```python
from build123d import *

# Parameters (mm, degrees)
BOSS_EXTRUDE1_DEPTH = 100
SKETCH2_R           = 2.75
CUT_EXTRUDE1_DEPTH  = 100
CUT_EXTRUDE2_DEPTH  = 100


with BuildPart() as part:
    # Sketch1 → Boss-Extrude1 (new body)
    with BuildSketch(Plane.XY):
        Polygon((0, 0), (-60, 0), (-60, -50), (-57, -50), (-57, -3), (0, -3), align=None)
    extrude(amount=BOSS_EXTRUDE1_DEPTH)

    # Sketch2 → Cut-Extrude1 (cut)
    with BuildSketch(Plane(origin=(0, 0, 0), x_dir=(1, 0, 0), z_dir=(0, 1, 0))):
        with Locations(Location((-11.813466521, -80.5, 0), (0, 0, 180))):
            Circle(SKETCH2_R)
        with Locations(Location((-48.186533479, -80.5, 0), (0, 0, 180))):
            Circle(SKETCH2_R)
        with Locations(Location((-30, -49, 0), (0, 0, 180))):
            Circle(SKETCH2_R)
    extrude(amount=-CUT_EXTRUDE1_DEPTH, mode=Mode.SUBTRACT)

    # Sketch3 → Cut-Extrude2 (cut)
    with BuildSketch(Plane(origin=(-57, 0, 0), x_dir=(0, 0, -1), z_dir=(1, 0, 0))):
        with BuildLine():
            Line((-80, -14), (-20, -14))
            ThreePointArc((-20, -14), (-16, -18), (-20, -22))
            Line((-20, -22), (-80, -22))
            ThreePointArc((-80, -22), (-84, -18), (-80, -14))
        make_face()
        with BuildLine():
            Line((-80, -39), (-20, -39))
            ThreePointArc((-20, -39), (-16, -35), (-20, -31))
            Line((-20, -31), (-80, -31))
            ThreePointArc((-80, -31), (-84, -35), (-80, -39))
        make_face()
    extrude(amount=-CUT_EXTRUDE2_DEPTH, mode=Mode.SUBTRACT)


solid = part.part
```
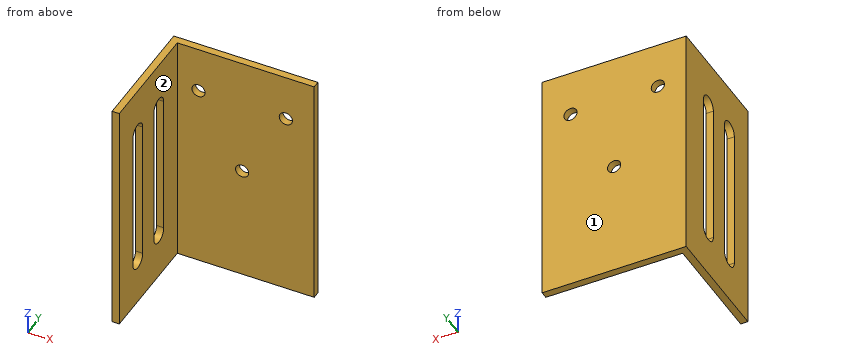
Geometry: final body of the model. Coordinates: model frame, mm. Face numbers are marked on the shaded views. A direction names the side the tool comes from. Give positions to 0.01 mm unless a question says otherwise; leave off trailing zeros. Loops run counter-clockwise (first coordinate to the right, second up) from the corner with the lowest first, then second, coordinate; pieces in that order, holes last. Notation, with made-up numbers: (61, 54) -> (90, 54) arc R27 ccw to (90, 92) -> close; hole circle Ø6 at (66, -12.75). An arc over 180 degrees is marked (long way). Use one line per item in the form item = value.
Item 1: Line query: probe 1 along Y at (x, z) = (-29, 23.5); probe 2 along X at (y, z) = (-40, 84); probe 3 along X at (y, z) = (-2, 80). Output: solid intervals per line, ascending.
A:
probe_1 = -3 to 0
probe_2 = -60 to -57
probe_3 = -60 to -50.89, -45.48 to -14.52, -9.11 to 0
Item 2: Access query for the marked faces 1 and 2. Directions: +Z, -Z, +X, -X, +Y, -Y. A direction counts if a zero-diameter tool reaches every point of the face in a straight line with its end or side. Return the directions, or none.
A:
face_1 = +Z, -Z, +X, -X, +Y
face_2 = +Z, -Z, +X, -Y
Item 3: Pin query (flat end, axial travel): P1, Ø4, axis at y = -43.5, z = 63.5, coming from the +X side; P2, Ø6.5, axis at x = -48.19, z = 80.5, coming from the -Y side. Return the tip coordinate at first contact, or that it passes through.
A:
P1 = -57
P2 = -3
Item 4: Section query D-D on z = 88. Output: boundary loops of the cut face in (x, y), and give its area (3 significant figures).
A:
outline = (-60, -50) -> (-57, -50) -> (-57, -3) -> (0, -3) -> (0, 0) -> (-60, 0) -> close
area = 321 mm^2
Item 5: Section query B-B on x = -30. Output: boundary loops of the cut face in (y, z), and give its area (4 significant figures).
A:
outline = (-3, 0) -> (0, 0) -> (0, 46.25) -> (-3, 46.25) -> close; (-3, 51.75) -> (0, 51.75) -> (0, 100) -> (-3, 100) -> close
area = 283.5 mm^2
Item 6: Section query A-A on z = 57.5. Output: boundary loops of the cut face in (x, y).
A:
outline = (-60, -50) -> (-57, -50) -> (-57, -39) -> (-60, -39) -> close; (-60, -31) -> (-57, -31) -> (-57, -22) -> (-60, -22) -> close; (-60, -14) -> (-57, -14) -> (-57, -3) -> (0, -3) -> (0, 0) -> (-60, 0) -> close
Item 7: Section query C-C on y = -18. Output: boundary loops of the cut face in (x, z).
A:
outline = (-60, 0) -> (-57, 0) -> (-57, 16) -> (-60, 16) -> close; (-60, 84) -> (-57, 84) -> (-57, 100) -> (-60, 100) -> close
